Source: CAD feature listing. Evaluate the final solid. Frame: model axes, mm. Coordinates: 2 decimals unless noted, no trailing zeros. Loops run counter-clockwise (first coordinate to the right, second up) from the corner with the lowest first, then second, coordinate; pieces in that order, holes last. Notation, with made-up numbers: (-36, 18) -> (-13, 18) arc R17 cw to (-13, 24) -> close; hole circle Ø11 at (-7, 62). An arc over 180 degrees is marked (long way). One line per question, with ' | ' between items. Start each with the question number.
```python
from build123d import *

# Parameters (mm, degrees)
SKETCH_2_R      = 60
SKETCH_2_R_2    = 2
SKETCH_2_R_3    = 1.5
SKETCH_2_R_4    = 3
EXTRUDE_1_DEPTH = 2


with BuildPart() as part:
    # 草图2 → 凸台-拉伸1 (new body)
    with BuildSketch(Plane.XY):
        with Locations((1.687240704, 17.758147453)):
            Circle(SKETCH_2_R)
        with Locations((-3.312759296, 32.050802338)):
            Circle(SKETCH_2_R_2, mode=Mode.SUBTRACT)
        with Locations((6.687240704, -16.249197662)):
            Circle(SKETCH_2_R_2, mode=Mode.SUBTRACT)
        with Locations((-3.312759296, -16.249197662)):
            Circle(SKETCH_2_R_2, mode=Mode.SUBTRACT)
        with Locations((-28.312759296, 32.758147453)):
            Circle(SKETCH_2_R_3, mode=Mode.SUBTRACT)
        with Locations((-52.312759296, 32.758147453)):
            Circle(SKETCH_2_R_3, mode=Mode.SUBTRACT)
        with Locations((-28.312759296, 2.758147453)):
            Circle(SKETCH_2_R_3, mode=Mode.SUBTRACT)
        with Locations((-52.312759296, 2.758147453)):
            Circle(SKETCH_2_R_3, mode=Mode.SUBTRACT)
        with Locations((31.687240704, 32.758147453)):
            Circle(SKETCH_2_R_3, mode=Mode.SUBTRACT)
        with Locations((55.687240704, 32.758147453)):
            Circle(SKETCH_2_R_3, mode=Mode.SUBTRACT)
        with Locations((31.687240704, 2.758147453)):
            Circle(SKETCH_2_R_3, mode=Mode.SUBTRACT)
        with Locations((55.687240704, 2.758147453)):
            Circle(SKETCH_2_R_3, mode=Mode.SUBTRACT)
        with Locations((36.689026372, -17.243638216)):
            Circle(SKETCH_2_R_2, mode=Mode.SUBTRACT)
        with Locations((-33.314544965, -17.243638216)):
            Circle(SKETCH_2_R_2, mode=Mode.SUBTRACT)
        with Locations((-33.314544965, 52.759933122)):
            Circle(SKETCH_2_R_2, mode=Mode.SUBTRACT)
        with Locations((36.689026372, 52.759933122)):
            Circle(SKETCH_2_R_2, mode=Mode.SUBTRACT)
        with Locations((-12.312759296, -3.241852547)):
            Circle(SKETCH_2_R_3, mode=Mode.SUBTRACT)
        with Locations((15.687240704, -3.241852547)):
            Circle(SKETCH_2_R_3, mode=Mode.SUBTRACT)
        with Locations((42.687240704, 24.758147453)):
            Circle(SKETCH_2_R_3, mode=Mode.SUBTRACT)
        with Locations((42.687240704, 10.758147453)):
            Circle(SKETCH_2_R_3, mode=Mode.SUBTRACT)
        with Locations((35.687240704, 17.758147453)):
            Circle(SKETCH_2_R_3, mode=Mode.SUBTRACT)
        with Locations((-39.312759296, 24.758147453)):
            Circle(SKETCH_2_R_3, mode=Mode.SUBTRACT)
        with Locations((-39.312759296, 10.758147453)):
            Circle(SKETCH_2_R_3, mode=Mode.SUBTRACT)
        with Locations((-32.312759296, 17.758147453)):
            Circle(SKETCH_2_R_3, mode=Mode.SUBTRACT)
        with Locations((1.687240704, -35.241852547)):
            Circle(SKETCH_2_R_3, mode=Mode.SUBTRACT)
        with Locations((6.687240704, 32.050802338)):
            Circle(SKETCH_2_R_2, mode=Mode.SUBTRACT)
        with Locations((1.687240704, -28.241852547)):
            Circle(SKETCH_2_R_4, mode=Mode.SUBTRACT)
        with Locations((8.687240704, -28.241852547)):
            Circle(SKETCH_2_R_3, mode=Mode.SUBTRACT)
        with Locations((-5.312759296, -28.241852547)):
            Circle(SKETCH_2_R_3, mode=Mode.SUBTRACT)
        with Locations((49.687240704, 10.758147453)):
            Circle(SKETCH_2_R_3, mode=Mode.SUBTRACT)
        with Locations((42.687240704, 17.758147453)):
            Circle(SKETCH_2_R_3, mode=Mode.SUBTRACT)
        with Locations((49.687240704, 24.758147453)):
            Circle(SKETCH_2_R_3, mode=Mode.SUBTRACT)
        with Locations((-39.312759296, 17.758147453)):
            Circle(SKETCH_2_R_3, mode=Mode.SUBTRACT)
        with Locations((-46.312759296, 10.758147453)):
            Circle(SKETCH_2_R_3, mode=Mode.SUBTRACT)
        with Locations((-46.312759296, 24.758147453)):
            Circle(SKETCH_2_R_3, mode=Mode.SUBTRACT)
        with Locations((1.687240704, 70.758147453)):
            Circle(SKETCH_2_R_3, mode=Mode.SUBTRACT)
        with Locations((1.687240704, 56.758147453)):
            Circle(SKETCH_2_R_3, mode=Mode.SUBTRACT)
        Polygon((1.037240704, -12.244197662), (1.037240704, -20.244197662), (2.337240704, -20.244197662), (2.337240704, -12.244197662), (11.646691261, -12.244197662), (11.646691261, 28.055802338), (2.337240704, 28.055802338), (2.337240704, 36.055802338), (1.037240704, 36.055802338), (1.037240704, 28.055802338), (-8.272209854, 28.055802338), (-8.272209854, -12.244197662), align=None, mode=Mode.SUBTRACT)
        with BuildLine():
            Line((14.187240704, 13.758147453), (14.187240704, 7.758147453))
            ThreePointArc((14.187240704, 7.758147453), (15.687240704, 6.258147453), (17.187240704, 7.758147453))
            Line((17.187240704, 7.758147453), (17.187240704, 13.758147453))
            ThreePointArc((17.187240704, 13.758147453), (15.687240704, 15.258147453), (14.187240704, 13.758147453))
        make_face(mode=Mode.SUBTRACT)
        with BuildLine():
            Line((-10.812759296, 7.758147453), (-10.812759296, 13.758147453))
            ThreePointArc((-10.812759296, 13.758147453), (-12.312759296, 15.258147453), (-13.812759296, 13.758147453))
            Line((-13.812759296, 13.758147453), (-13.812759296, 7.758147453))
            ThreePointArc((-13.812759296, 7.758147453), (-12.312759296, 6.258147453), (-10.812759296, 7.758147453))
        make_face(mode=Mode.SUBTRACT)
        with BuildLine():
            Line((-10.812759296, 21.758147453), (-10.812759296, 27.758147453))
            ThreePointArc((-10.812759296, 27.758147453), (-12.312759296, 29.258147453), (-13.812759296, 27.758147453))
            Line((-13.812759296, 27.758147453), (-13.812759296, 21.758147453))
            ThreePointArc((-13.812759296, 21.758147453), (-12.312759296, 20.258147453), (-10.812759296, 21.758147453))
        make_face(mode=Mode.SUBTRACT)
        with BuildLine():
            Line((17.187240704, 21.758147453), (17.187240704, 27.758147453))
            ThreePointArc((17.187240704, 27.758147453), (15.687240704, 29.258147453), (14.187240704, 27.758147453))
            Line((14.187240704, 27.758147453), (14.187240704, 21.758147453))
            ThreePointArc((14.187240704, 21.758147453), (15.687240704, 20.258147453), (17.187240704, 21.758147453))
        make_face(mode=Mode.SUBTRACT)
        with BuildLine():
            Line((15.687240704, -29.741852547), (22.687240704, -29.741852547))
            ThreePointArc((22.687240704, -29.741852547), (24.187240704, -28.241852547), (22.687240704, -26.741852547))
            Line((22.687240704, -26.741852547), (15.687240704, -26.741852547))
            ThreePointArc((15.687240704, -26.741852547), (14.187240704, -28.241852547), (15.687240704, -29.741852547))
        make_face(mode=Mode.SUBTRACT)
        with BuildLine():
            Line((-19.312759296, -29.741852547), (-12.312759296, -29.741852547))
            ThreePointArc((-12.312759296, -29.741852547), (-10.812759296, -28.241852547), (-12.312759296, -26.741852547))
            Line((-12.312759296, -26.741852547), (-19.312759296, -26.741852547))
            ThreePointArc((-19.312759296, -26.741852547), (-20.812759296, -28.241852547), (-19.312759296, -29.741852547))
        make_face(mode=Mode.SUBTRACT)
        with BuildLine():
            Line((-19.312759296, 62.258147453), (-12.312759296, 62.258147453))
            ThreePointArc((-12.312759296, 62.258147453), (-10.812759296, 63.758147453), (-12.312759296, 65.258147453))
            Line((-12.312759296, 65.258147453), (-19.312759296, 65.258147453))
            ThreePointArc((-19.312759296, 65.258147453), (-20.812759296, 63.758147453), (-19.312759296, 62.258147453))
        make_face(mode=Mode.SUBTRACT)
        with BuildLine():
            Line((15.687240704, 62.258147453), (22.687240704, 62.258147453))
            ThreePointArc((22.687240704, 62.258147453), (24.187240704, 63.758147453), (22.687240704, 65.258147453))
            Line((22.687240704, 65.258147453), (15.687240704, 65.258147453))
            ThreePointArc((15.687240704, 65.258147453), (14.187240704, 63.758147453), (15.687240704, 62.258147453))
        make_face(mode=Mode.SUBTRACT)
        with BuildLine():
            Line((-19.312759296, 37.258147453), (-12.312759296, 37.258147453))
            ThreePointArc((-12.312759296, 37.258147453), (-10.812759296, 38.758147453), (-12.312759296, 40.258147453))
            Line((-12.312759296, 40.258147453), (-19.312759296, 40.258147453))
            ThreePointArc((-19.312759296, 40.258147453), (-20.812759296, 38.758147453), (-19.312759296, 37.258147453))
        make_face(mode=Mode.SUBTRACT)
        with BuildLine():
            Line((15.687240704, 37.258147453), (22.687240704, 37.258147453))
            ThreePointArc((22.687240704, 37.258147453), (24.187240704, 38.758147453), (22.687240704, 40.258147453))
            Line((22.687240704, 40.258147453), (15.687240704, 40.258147453))
            ThreePointArc((15.687240704, 40.258147453), (14.187240704, 38.758147453), (15.687240704, 37.258147453))
        make_face(mode=Mode.SUBTRACT)
        with BuildLine():
            Line((49.687240704, 16.258147453), (55.687240704, 16.258147453))
            ThreePointArc((55.687240704, 16.258147453), (57.187240704, 17.758147453), (55.687240704, 19.258147453))
            Line((55.687240704, 19.258147453), (49.687240704, 19.258147453))
            ThreePointArc((49.687240704, 19.258147453), (48.187240704, 17.758147453), (49.687240704, 16.258147453))
        make_face(mode=Mode.SUBTRACT)
        with BuildLine():
            Line((-52.312759296, 16.258147453), (-46.312759296, 16.258147453))
            ThreePointArc((-46.312759296, 16.258147453), (-44.812759296, 17.758147453), (-46.312759296, 19.258147453))
            Line((-46.312759296, 19.258147453), (-52.312759296, 19.258147453))
            ThreePointArc((-52.312759296, 19.258147453), (-53.812759296, 17.758147453), (-52.312759296, 16.258147453))
        make_face(mode=Mode.SUBTRACT)
        with BuildLine():
            Line((-5.312759296, 62.258147453), (8.687240704, 62.258147453))
            ThreePointArc((8.687240704, 62.258147453), (10.187240704, 63.758147453), (8.687240704, 65.258147453))
            Line((8.687240704, 65.258147453), (-5.312759296, 65.258147453))
            ThreePointArc((-5.312759296, 65.258147453), (-6.812759296, 63.758147453), (-5.312759296, 62.258147453))
        make_face(mode=Mode.SUBTRACT)
    extrude(amount=EXTRUDE_1_DEPTH)


solid = part.part
```
(1) Ray query, L1, parallel to Y at x = 19.5, z = 1.6; L2, parallel to Y at x = 18, z = 0.2; L3, parallel to X at y = 53, z = 0.3. Return the intervals inside material, ascending.
(2) Cut plane A-A, the plane x = 20.5. Return the cut outline in (y, z), and give its area (3 significant figures).
(3) Contact query for flat-ended pins moving along their axis: pin 1 Ø2.5 at (x, y) = (31.69, 32.76) entering from -Z; pin 2 Ø1 at (x, z) = (0, 1) entering from -Y; pin 3 Ø1 at (y, z) = (51.5, 2) entering from +X; pin 4 Ø1 at (x, z) = (-2.5, 1) entering from -Y. Output: stop coordinate, or through.
(4) Draft query along Y for faces 1 (the cylindrical face through (1.297, -25.267, 0.986)), 2 (the cylindrical face through (41.58, 25.77, 0.99)), 3 (the cylindrical face through (57.112, -5.222, 0.986)). Return one class per face: pulls with the +Y half, pulls with the -Y half, needs draft (parallel to the pull), parting line crosses it, or undercut.
(5) Cut plane B-B, the plane z = 0.7. State how many separate pieces and enclosed holes the cut face has, and give its area (3 significant figures).
Here are the results:
1) L1: y = -39.54 to -29.74, -26.74 to 37.26, 40.26 to 62.26, 65.26 to 75.05 | L2: y = -39.98 to -29.74, -26.74 to 37.26, 40.26 to 62.26, 65.26 to 75.5 | L3: x = -46.87 to -35.3, -31.33 to 34.7, 38.67 to 50.25
2) outline: (-39.22, 0) -> (-29.74, 0) -> (-29.74, 2) -> (-39.22, 2) -> close; (-26.74, 0) -> (37.26, 0) -> (37.26, 2) -> (-26.74, 2) -> close; (40.26, 0) -> (62.26, 0) -> (62.26, 2) -> (40.26, 2) -> close; (65.26, 0) -> (74.73, 0) -> (74.73, 2) -> (65.26, 2) -> close | area: 210 mm2
3) pin 1: passes through | pin 2: stops at y = -42.23 | pin 3: stops at x = 51.64 | pin 4: stops at y = -42.13
4) face 1: undercut | face 2: undercut | face 3: parting line crosses it
5) separate pieces: 1 | enclosed holes: 50 | area: 9,800 mm2
